from build123d import *

# Parameters (mm, degrees)
SKETCH1_R               = 32.5
BOSS_EXTRUDE1_DEPTH     = 100
SKETCH2_R               = 50
BOSS_EXTRUDE2_DEPTH     = 400
BOSS_EXTRUDE3_DEPTH     = 50
SKETCH7_R               = 10
CUT_EXTRUDE2_DEPTH      = 1
CUT_EXTRUDE2_DEPTH_BACK = 141


with BuildPart() as part:
    # Sketch1 → Boss-Extrude1 (new body)
    with BuildSketch(Plane(origin=(0, 0, 0), x_dir=(1, 0, 0), z_dir=(0, 1, 0))):
        Circle(SKETCH1_R)
    extrude(amount=BOSS_EXTRUDE1_DEPTH)

    # Sketch2 → Boss-Extrude2 (add)
    with BuildSketch(Plane(origin=(0, 100, 0), x_dir=(1, 0, 0), z_dir=(0, 1, 0))):
        Circle(SKETCH2_R)
    extrude(amount=BOSS_EXTRUDE2_DEPTH)

    # Sketch6 → Boss-Extrude3 (add, symmetric)
    with BuildSketch(Plane(origin=(0, 0, 0), x_dir=(0, 0, -1), z_dir=(1, 0, 0))):
        Polygon((-50, 500), (-60, 510), (-60, 600), (-70, 600), (-70, 505.857864376), (-50, 485.857864376), (50, 485.857864376), (70, 505.857864376), (70, 600), (60, 600), (60, 510), (50, 500), align=None)
    extrude(amount=BOSS_EXTRUDE3_DEPTH, both=True)

    # Sketch7 → Cut-Extrude2 (cut, two sides)
    with BuildSketch(Plane.XY.offset(70)) as cut_extrude2_sk:
        with Locations((0, 550)):
            Circle(SKETCH7_R)
        with BuildLine():
            Line((-50, 550), (-50, 605))
            Line((-50, 605), (50, 605))
            Line((50, 605), (50, 550))
            ThreePointArc((50, 550), (0, 600), (-50, 550))
        make_face()
    extrude(amount=CUT_EXTRUDE2_DEPTH, mode=Mode.SUBTRACT)
    extrude(cut_extrude2_sk.sketch, amount=-CUT_EXTRUDE2_DEPTH_BACK, mode=Mode.SUBTRACT)


solid = part.part
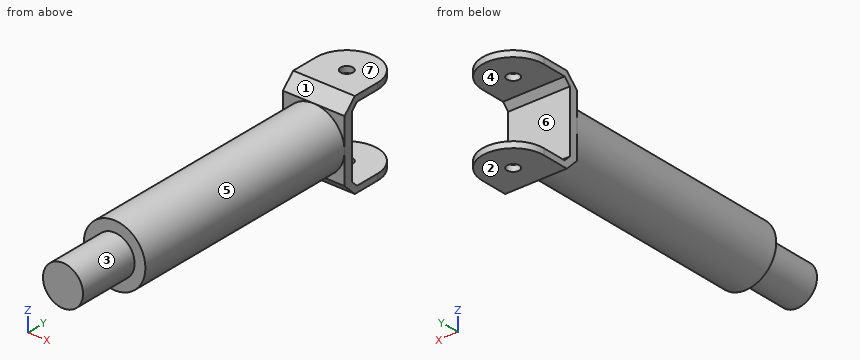
For this review, take the finished solid that the model builds, in its own axes (mm). Face numbers are marked on the shaded views. A direction names the side the tool comes from. Coordinates: 2 decimals unless noted, no trailing zeros. Order: outer loops, then holes, each group sorted by start corner. A loop starts at its lowest first (then second) coordinate and runs counter-clockwise, first axis right, second up. Notation, with made-up numbers: (-35.5, 79.25) - (-0.5, 79.25) arc R27 ccw to (-0.5, 113.25) - close; hole circle Ø6 at (8.25, -1). An arc over 180 degrees is marked (long way). Use one line per item in the form item = value.
Q1. Draft analysis for pull direction Z (two halves, no side actions). For the marked faces 1, 2, 3 and 4, state which applies: +Z half, -Z half, draft (parallel to the pull), parting line (faces both ways), or undercut.
Checked values:
face_1 = +Z half
face_2 = -Z half
face_3 = parting line
face_4 = undercut
Q2. Consider section A-A (z = -38). Give the boundary of the cut face in (x, y), then the cut area to 3 significant figures.
Checked values:
outline = (-50, 485.86) - (-32.5, 485.86) - (-32.5, 100) - (32.5, 100) - (32.5, 485.86) - (50, 485.86) - (50, 500) - (-50, 500) - close
area = 26,500 mm2
Q3. For the marked faces 5, 6 and 7, list the 3-axis set-ups (+Z, -Z, +X, -X, +Y, -Y) from which the entire face can be reached by the end or side of a thin tool; tool diameter is ignored.
Checked values:
face_5 = -Y
face_6 = +X, -X, +Y
face_7 = +Z, +X, -X, +Y, -Y
Q4. Consider section B-B (x = 40.5). Give the boundary of the cut face in (y, z), then the cut area to 3 significant figures.
Checked values:
outline = (100, -29.32) - (485.86, -29.32) - (485.86, -50) - (505.86, -70) - (579.32, -70) - (579.32, -60) - (510, -60) - (500, -50) - (500, 50) - (510, 60) - (579.32, 60) - (579.32, 70) - (505.86, 70) - (485.86, 50) - (485.86, 29.32) - (100, 29.32) - close
area = 25,900 mm2
Q5. For P1, Ø5, axis at x = -26.5, z = -5.5, coming from the +Y side; P2, Ø8, axis at x = -10, y = 226, coming from the -Z side; P3, Ø3, axis at y = 158, z = -28.5, coming from the -X side; P4, Ø18, axis at x = 0, y = 550, coming from the -Z side, all flat-tipped, find the tip position at first contact; note any pin that passes through.
Checked values:
P1 = 500
P2 = -49.64
P3 = -42.08
P4 = through
Q6. For probe 1 along X at (y, z) = (550, 68); probe 2 along Z at (x, y) = (42.5, 536.5); probe 3 along Y at (x, z) = (10, -15), list the stretches that pass through material, from the lowest coordinate up. Write a range as from..to.
Checked values:
probe_1 = -50..-10, 10..50
probe_2 = -70..-60, 60..70
probe_3 = 0..500
Q7. Consider section C-C (y = 321). Give the boundary of the cut face in (x, z), then the cut area to 3 significant figures.
Checked values:
outline = circle Ø100 at (0, 0)
area = 7,850 mm2
